Here's how the part is built. I have some questions about the finished solid (model axes, mm). A direction names the side the tool comes from. Round coordinates to 2 decimals unless told otherwise and drop trailing zeros. Loops run counter-clockwise (first coordinate to the right, second up) from the corner with the lowest first, then second, coordinate; pieces in that order, holes last. Notation, with made-up numbers: M 2.25,49.25 L 21.25,49.25 A23 cw 21.25,61.25 Z; hole C -31.75,58 d3. An arc over 180 degrees is marked long. Answer as a JSON object with one key per item and string values.
from build123d import *

# Parameters (mm, degrees)
SKETCH_1_R          = 11
EXTRUDE_1_DEPTH     = 2.5
SKETCH_2_R          = 5
EXTRUDE_2_DEPTH     = 8
CUT_EXTRUDE_1_REACH = 20.768
SKETCH_3_R          = 2.5
CUT_EXTRUDE_2_REACH = 19.493
SKETCH_4_R          = 1.5


with BuildPart() as part:
    # 草图1 → 凸台-拉伸1 (new body)
    with BuildSketch(Plane.XY):
        Circle(SKETCH_1_R)
    extrude(amount=EXTRUDE_1_DEPTH)

    # 草图2 → 凸台-拉伸2 (add)
    with BuildSketch(Plane.XY.offset(2.5)):
        Circle(SKETCH_2_R)
    extrude(amount=EXTRUDE_2_DEPTH)

    # 草图3 → 切除-拉伸1 (cut, up to next)
    with BuildSketch(Plane.XY.offset(10.5), mode=Mode.PRIVATE) as cut_extrude_1_sk1:
        Circle(SKETCH_3_R)
    cut_extrude_1_tool1 = extrude(cut_extrude_1_sk1.sketch, amount=-CUT_EXTRUDE_1_REACH, mode=Mode.PRIVATE) & part.part
    add(cut_extrude_1_tool1.solids().sort_by_distance((0, 0, 10.5))[0], mode=Mode.SUBTRACT)

    # 草图4 → 切除-拉伸2 (cut, up to next)
    with BuildSketch(Plane.XY.offset(2.5), mode=Mode.PRIVATE) as cut_extrude_2_sk1:
        with Locations((8, 0)):
            Circle(SKETCH_4_R)
    cut_extrude_2_tool1 = extrude(cut_extrude_2_sk1.sketch, amount=-CUT_EXTRUDE_2_REACH, mode=Mode.PRIVATE) & part.part
    # 草图4 → 切除-拉伸2 (cut, up to next)
    with BuildSketch(Plane.XY.offset(2.5), mode=Mode.PRIVATE) as cut_extrude_2_sk2:
        with Locations((0, -8)):
            Circle(SKETCH_4_R)
    cut_extrude_2_tool2 = extrude(cut_extrude_2_sk2.sketch, amount=-CUT_EXTRUDE_2_REACH, mode=Mode.PRIVATE) & part.part
    # 草图4 → 切除-拉伸2 (cut, up to next)
    with BuildSketch(Plane.XY.offset(2.5), mode=Mode.PRIVATE) as cut_extrude_2_sk3:
        with Locations((-8, 0)):
            Circle(SKETCH_4_R)
    cut_extrude_2_tool3 = extrude(cut_extrude_2_sk3.sketch, amount=-CUT_EXTRUDE_2_REACH, mode=Mode.PRIVATE) & part.part
    # 草图4 → 切除-拉伸2 (cut, up to next)
    with BuildSketch(Plane.XY.offset(2.5), mode=Mode.PRIVATE) as cut_extrude_2_sk4:
        with Locations((0, 8)):
            Circle(SKETCH_4_R)
    cut_extrude_2_tool4 = extrude(cut_extrude_2_sk4.sketch, amount=-CUT_EXTRUDE_2_REACH, mode=Mode.PRIVATE) & part.part
    add(cut_extrude_2_tool1.solids().sort_by_distance((8, 0, 2.5))[0], mode=Mode.SUBTRACT)
    add(cut_extrude_2_tool2.solids().sort_by_distance((0, -8, 2.5))[0], mode=Mode.SUBTRACT)
    add(cut_extrude_2_tool3.solids().sort_by_distance((-8, 0, 2.5))[0], mode=Mode.SUBTRACT)
    add(cut_extrude_2_tool4.solids().sort_by_distance((0, 8, 2.5))[0], mode=Mode.SUBTRACT)


solid = part.part
Item 1: I'm going to push flat-ended pins straight in: pin 1 Ø5 at (x, z) = (-6, 9) entering from -Y; pin 2 Ø2 at (y, z) = (4.5, 9) entering from -X; pin 3 Ø1.5 at (x, y) = (-6.5, -7.5) entering from +Z. Where does each tip first touch, or does it pass through?
Resolved:
{"pin 1": "y = -3.57", "pin 2": "x = -3.57", "pin 3": "z = 2.5"}
Item 2: If we mould it in two halves opening along Y, with no side actions, what happens to faces 1 (the face through (2, -2, 10.5)), 2 (the face through (6.5, 0.07, 1.27)), 3 (the face through (-2.38, -10.74, 1.23)), 4 (the face through (-9.5, 0.07, 1.27))? For each: pulls with the +Y half, pulls with the -Y half, needs draft (parallel to the pull), parting line crosses it, or undercut.
Resolved:
{"face 1": "needs draft", "face 2": "undercut", "face 3": "parting line crosses it", "face 4": "undercut"}
Item 3: Please list where these lines run through material, in increasing order: probe 1 along Y at (x, z) = (0, 1.65); probe 2 along X at (y, z) = (-1.25, 2.25); probe 3 along Y at (x, z) = (0, 6.75). Write a range as from..to.
Resolved:
{"probe 1": "-11..-9.5, -6.5..-2.5, 2.5..6.5, 9.5..11", "probe 2": "-10.93..-8.83, -7.17..-2.17, 2.17..7.17, 8.83..10.93", "probe 3": "-5..-2.5, 2.5..5"}
Item 4: I want a section at C-C, the plane z = 0.5. Please give me the cut outline in (x, y), then the cut area to 3 significant figures.
Resolved:
{"outline": "C 0,0 d22; hole C -8,0 d3; hole C 0,0 d5; hole C 0,-8 d3; hole C 0,8 d3; hole C 8,0 d3", "area": "332 mm²"}
Item 5: I want a section at A-A, the plane y = 0. Please give me the cut outline in (x, z), then the cut area to 3 significant figures.
Resolved:
{"outline": "M -11,0 L -9.5,0 L -9.5,2.5 L -11,2.5 Z; M -6.5,0 L -2.5,0 L -2.5,10.5 L -5,10.5 L -5,2.5 L -6.5,2.5 Z; M 2.5,0 L 6.5,0 L 6.5,2.5 L 5,2.5 L 5,10.5 L 2.5,10.5 Z; M 9.5,0 L 11,0 L 11,2.5 L 9.5,2.5 Z", "area": "67.5 mm²"}
Item 6: I want a section at D-D, the plane y = -7.5. Please give me the cut outline in (x, z), then the cut area to 3 significant figures.
Resolved:
{"outline": "M -8.05,0 L -1.41,0 L -1.41,2.5 L -8.05,2.5 Z; M 1.41,0 L 8.05,0 L 8.05,2.5 L 1.41,2.5 Z", "area": "33.2 mm²"}
Item 7: On a 3-axis mill with a long thin cutter (end or side, diameter ignored), from which of +Z, -Z, +X, -X, +Y, -Y can I reach the whole of each face in a straight line? I mean faces 5 (the face through (-0.325, 6.536, 1.268)), 6 (the face through (5, -2, 2.5)). Say none if no direction works.
Resolved:
{"face 5": "+Z, -Z", "face 6": "+Z"}
